Can you work these out from the model? Positions are in its coordinate system, mm. Face numbers are marked on the shaded views. A direction names the side the tool comes from. Coordinates: 2 decimals unless noted, no trailing zeros.
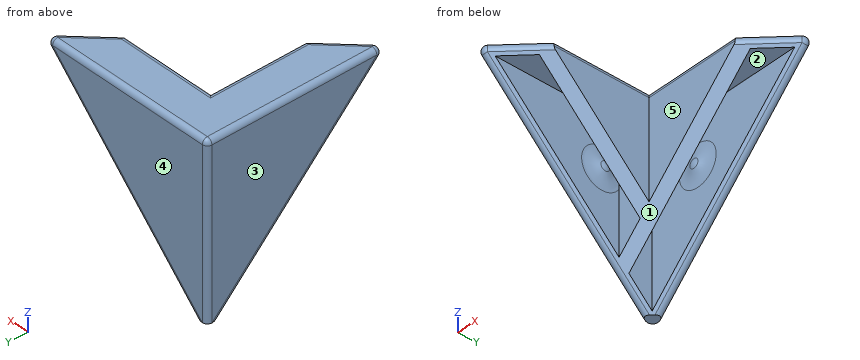
```python
from build123d import *

# Parameters (mm, degrees)
F1_DEPTH  = 28.575
F3_R      = 38.1
F4_DEPTH  = 32.9965678842
F6_W      = 26.9748
F6_H      = 3.5145800794
F6_W_2    = 3.5145800794
F6_H_2    = 21.971
F7_DEPTH  = 26.9758
F8_R      = 0.762
F15_W     = 1.8396307345
F15_H     = 1.8396307345
F16_DEPTH = 26.4941772846


# Not quite as in the source:
# - a fillet or chamfer that OpenCascade refuses, or shapes differently, is made with other operations: its cross-section is extruded or revolved along the edge and cut away or added
# - a pattern or mirror of a feature is missing from the dataset's text; its kind, count and spacing are read off the source's solid


with BuildPart() as f1:
    # F0 (on Top) → F1 (new body)
    with BuildSketch(Plane.XY):
        Polygon((0, -21.971), (0, 0), (21.971, 0), (21.971, 6.604), (-6.604, 6.604), (-6.604, -21.971), align=None)
    extrude(amount=-F1_DEPTH)

    # F3 (on 3pt) → F4 (cut, through all)
    with BuildSketch(Plane(origin=(5.1223333333, -5.1223333333, -5.1223333333), x_dir=(0.8164965809, 0.4082482905, 0.4082482905), z_dir=(0.5773502692, -0.5773502692, -0.5773502692))):
        Circle(F3_R)
    extrude(amount=F4_DEPTH, mode=Mode.SUBTRACT)

    # F6 (on offset) → F7 (cut, through all)
    with BuildSketch(Plane.XY.offset(-1.6002)):
        with Locations((8.4836, 3.2465099603)):
            Rectangle(F6_W, F6_H)
        with Locations((-3.2465099603, -10.9855)):
            Rectangle(F6_W_2, F6_H_2)
    extrude(amount=-F7_DEPTH, mode=Mode.SUBTRACT)

    # F8
    f8_edges = [f1.edges().sort_by_distance(p)[0] for p in [
        (7.6835, 6.604, 0),
        (18.669, 3.302, 0),
        (7.6835, 0, 0),
        (0, -7.6835, 0),
        (-3.302, -18.669, 0),
        (-6.604, -7.6835, 0),
        (-6.604, 6.604, -14.2875),
        (7.6835, 6.604, -14.2875),
        (-6.604, -7.6835, -14.2875),
    ]]
    fillet(f8_edges, radius=F8_R)

    # F10 (on offset) → F11 (revolve)
    with BuildSketch(Plane.YZ.offset(2.6162)):
        with BuildLine():
            ThreePointArc((4.2418, -9.2202), (4.4469151823, -9.9607308906), (5.0038, -10.4902))
            Line((5.0038, -10.4902), (5.0038, -9.2202))
            Line((5.0038, -9.2202), (4.2418, -9.2202))
        make_face()
    f11 = revolve(axis=Axis((2.6162, 4.6228, -9.2202), (0, -1, 0)))

    # F11_copies: F11 across plane
    add(f11.mirror(Plane(origin=(0, 0, 0), x_dir=(0.7071067796, -0.7071067828, 0), z_dir=(-0.7071067828, -0.7071067796, 0))))

    # F14: fillet of radius 5.08 on 3 edges, made by hand

    # F14_s1 → F14_t2 (revolve)
    with BuildSketch(Plane.YZ.offset(2.6162)):
        with BuildLine():
            ThreePointArc((5.0038, -12.278765023), (4.853123865, -11.0506908258), (4.4100337662, -9.8954676025))
            ThreePointArc((4.4100337662, -9.8954676025), (4.662543942, -10.2371346569), (5.0038, -10.4902))
            Line((5.0038, -10.4902), (5.0038, -12.278765023))
        make_face()
    revolve(axis=Axis((2.6162, 5.0038, -9.2202), (0, -1, 0)))

    # F14_s3 → F14_t4 (revolve)
    with BuildSketch(Plane.XZ.offset(2.6161999777)):
        with BuildLine():
            ThreePointArc((-5.0038, -12.2787650011), (-4.8531238674, -11.0506908133), (-4.4100337753, -9.8954675976))
            ThreePointArc((-4.4100337753, -9.8954675976), (-4.6625439517, -10.237134655), (-5.0038000116, -10.4902))
            Line((-5.0038000116, -10.4902), (-5.0038, -12.2787650011))
        make_face()
    revolve(axis=Axis((-5.0038000116, -2.6161999777, -9.2202), (-1, 4.4e-09, 0)))

    # F15 (on face) → F16 (cut, through all)
    with BuildSketch(Plane(origin=(-6.604, 0, 0), x_dir=(0, -1, 0), z_dir=(-1, 0, 0))):
        with Locations((-5.6841846327, -26.6509926519)):
            Rectangle(F15_W, F15_H)
    extrude(amount=-F16_DEPTH, mode=Mode.SUBTRACT)


solid = f1.part
```
1. On a 3-axis mill with a long thin cutter (end or side, diameter ignored), from which of +Z, -Z, +X, -X, +Y, -Y can I reach the whole of each face in a straight line? I mean the marked faces 4 and 5. Say none if no direction works.
Completed:
face 4: +Z, -Z, +X, -X, +Y
face 5: +Z, -Z, +X, -Y
2. Thinking about a two-plate mould opening in Y: for the marked faces 1, 2 and 3, which applies, pulls with the +Y half, pulls with the -Y half, needs draft (parallel to the pull), parting line crosses it, or undercut?
Completed:
face 1: pulls with the -Y half
face 2: undercut
face 3: needs draft
3. Please list where these lines run through material, in increasing order: probe 1 along Y at (x, z) = (2.25, -13); probe 2 along X at (y, z) = (-1.75, -5); probe 3 along X at (y, z) = (4.5, -15.5).
Completed:
probe 1: y = 0 to 1.49, 5 to 6.6
probe 2: x = -6.6 to -5, -1.49 to 0
probe 3: x = -6.6 to -5
4. I'm going to push flat-ended pins straight in: pin 1 (1.1 mm diameter, centred on x = -3.5, y = -9, fed in from -Z); pin 2 (12 mm diameter, centred on x = 7, z = -10.5, fed in from -Y); pin 3 (4 mm diameter, centred on y = -1.5, z = -17, fed in from +X). Where does each tip first touch, or does it pass through?
Completed:
pin 1: stops at z = -1.6
pin 2: stops at y = 0
pin 3: stops at x = -0.3
